Read the model definition and answer for the solid it produces. Units are mm, in the model's axes. Face numbers are marked on the shaded views. A direction names the side the tool comes from. Coordinates: 2 decimals unless noted, no trailing zeros. Order: outer loops, then holes, each group sorted by start corner. A loop starts at its lowest first (then second) coordinate and runs counter-clockwise, first axis right, second up. Notation, with made-up numbers: (10, 21) -> (32, 21) arc R8 cw to (32, 33) -> close; hole circle Ø10 at (-16.75, -13.5). An arc over 180 degrees is marked (long way). Answer as a JSON object with one key per item and string values. Group by question number.
1) A tool of negligible diameter and unlimited length cuts with its end or side. For the marked faces 1, 2 and 3, from which of +Z, -Z, +X, -X, +Y, -Y can it reach the whole face along a straight path? Write none if from no direction.
2) Section D-D on y = 29.5 is taken. Determine the outline of the cut face in (x, z).
3) Given pin 1 (4 mm diameter, centred on x = 22.5, z = -23.5, fed in from +Y); pin 2 (1.5 mm diameter, centred on x = -4, y = 11.5, fed in from +Z); pin 3 (8 mm diameter, centred on x = -19.5, y = 25, fed in from +Z); pin 4 (1 mm diameter, centred on y = 9.5, z = -37.5, fed in from -X), each flat-ended and moving along its own axis, determine where each tip first touches the part or whether it passes through.
4) Section A-A on z = 0 is taken. Count the separate pieces of the cut face and the enclosed holes in it, and give its area (3 significant figures).
5) Section C-C on y = 60.5 is taken. Determine the outline of the cut face in (x, z).
6) Consider L1, parallel to Y at x = -18.5, z = 26; L2, parallel to X at y = 61, z = 1; L3, parallel to Z at x = 7.5, y = 12. Determine where each line is inside the solid, lowest interval first.
from build123d import *

# Parameters (mm, degrees)
F0_R     = 50
F0_R_2   = 5
F1_DEPTH = 8
F2_R     = 27
F3_DEPTH = 10
F4_R     = 22
F5_DEPTH = 32
F6_R     = 18
F7_DEPTH = 20
F8_R     = 22.5
F9_DEPTH = 8
F11_D    = 20
F12_SIZE = 2
F13_R    = 3
F14_SIZE = 1


with BuildPart() as f1:
    # F0 (on Front) → F1 (new body)
    with BuildSketch(Plane.XZ):
        Circle(F0_R)
        with Locations((-26.5165042945, -26.5165042945)):
            Circle(F0_R_2, mode=Mode.SUBTRACT)
        with Locations((0, -37.5)):
            Circle(F0_R_2, mode=Mode.SUBTRACT)
        with Locations((26.5165042945, -26.5165042945)):
            Circle(F0_R_2, mode=Mode.SUBTRACT)
        with Locations((-37.5, 0)):
            Circle(F0_R_2, mode=Mode.SUBTRACT)
        with Locations((-26.5165042945, 26.5165042945)):
            Circle(F0_R_2, mode=Mode.SUBTRACT)
        with Locations((37.5, 0)):
            Circle(F0_R_2, mode=Mode.SUBTRACT)
        with Locations((0, 37.5)):
            Circle(F0_R_2, mode=Mode.SUBTRACT)
        with Locations((26.5165042945, 26.5165042945)):
            Circle(F0_R_2, mode=Mode.SUBTRACT)
    extrude(amount=-F1_DEPTH)

    # F2 (on face) → F3 (join)
    with BuildSketch(Plane(origin=(0, 8, 0), x_dir=(-1, 0, 0), z_dir=(0, 1, 0))):
        Circle(F2_R)
    extrude(amount=F3_DEPTH)

    # F4 (on face) → F5 (join)
    with BuildSketch(Plane(origin=(0, 18, 0), x_dir=(-1, 0, 0), z_dir=(0, 1, 0))):
        Circle(F4_R)
    extrude(amount=F5_DEPTH)

    # F6 (on face) → F7 (join)
    with BuildSketch(Plane(origin=(0, 50, 0), x_dir=(-1, 0, 0), z_dir=(0, 1, 0))):
        Circle(F6_R)
    extrude(amount=F7_DEPTH)

    # F8 (on face) → F9 (cut)
    with BuildSketch(Plane.XZ):
        Circle(F8_R)
    extrude(amount=-F9_DEPTH, mode=Mode.SUBTRACT)

    # F11 (through all)
    with Locations(Plane.XZ.offset(-8)):
        with Locations((0, 0)):
            Hole(F11_D / 2)

    # F12
    f12_edges = [f1.edges().sort_by_distance(p)[0] for p in [
        (-22.5, 0, 0),
        (18, 70, 0),
    ]]
    chamfer(f12_edges, length=F12_SIZE)

    # F13
    f13_edges = [f1.edges().sort_by_distance(p)[0] for p in [
        (-22.5, 8, 0),
        (22, 18, 0),
        (18, 50, 0),
    ]]
    fillet(f13_edges, radius=F13_R)

    # F14
    f14_edges = [f1.edges().sort_by_distance(p)[0] for p in [
        (-50, 0, 0),
        (-50, 8, 0),
    ]]
    chamfer(f14_edges, length=F14_SIZE)


solid = f1.part
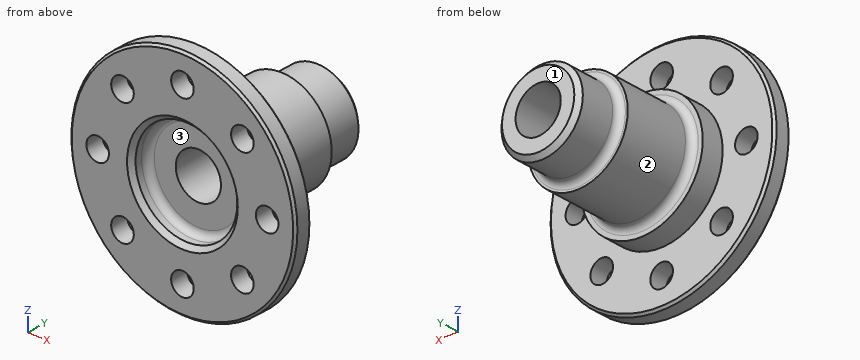
Worked answers:
{
 "1": {"face 1": "+Z, -Z, +X, -X, +Y", "face 2": "+Y", "face 3": "-Y"},
 "2": {"outline": "circle Ø44 at (0, 0); hole circle Ø20 at (0, 0)"},
 "3": {"pin 1": "stops at y = 8", "pin 2": "stops at z = 26.8", "pin 3": "stops at z = 15.61", "pin 4": "passes through"},
 "4": {"separate pieces": "4", "enclosed holes": "0", "area": "1,710 mm²"},
 "5": {"outline": "circle Ø36 at (0, 0); hole circle Ø20 at (0, 0)"},
 "6": {"L1": "y = 0 to 8", "L2": "x = -17.97 to -9.95, 9.95 to 17.97", "L3": "z = -25.94 to -6.61, 6.61 to 25.94"}
}
